Geometry check sheet. Reference: the model listing, model coordinates, mm. Coordinates: 2 decimals unless noted, no trailing zeros. Order: outer loops, then holes, each group sorted by start corner. A loop starts at its lowest first (then second) coordinate and runs counter-clockwise, first axis right, second up. Notation, with made-up numbers: (-33, 72.25) - (-13, 72.25) arc R16 ccw to (-13, 101.25) - close; hole circle Ø8 at (-6, 27). An arc over 180 degrees is marked (long way). Return JSON: item names as keys, results as strings. Group by question number.
Item 1: Scan lines: probe 1 along Y at (x, z) = (41, -2); probe 2 along Y at (x, z) = (-62, 0.25); probe 3 along X at (y, z) = (-2.5, 1.5). Record each from-to range of solid material in increasing order.
Item 2: Draft check along X on faces 1 (the conical face through (-23.88, -0.56, 4.27)), 2 (the conical face through (37.715, 3.943, 1.242)), 3 (the flat face through (-76.2, 0, 0)). Enter one of: pulls with the +X half, pulls with the -X half, needs draft (parallel to the pull), parting line crosses it, or undercut.
Item 3: Section check A-A on x = -63. Enter the section's corners in (y, z) (1 decimal).
Item 4: Gauge pin test, flat ends, axial feed: pin 1 (2 mm diameter, centred on x = 5, y = 2, fed in from +Z); pin 2 (2 mm diameter, centred on x = -4.5, z = -0.5, fed in from +Y); pin 3 (3 mm diameter, centred on y = -2.5, z = 3.5, fed in from +X). Record the tip position at first contact, or that the pin passes through.
Item 5: Section check B-B on x = 21. Enter the section's corners in (y, z) (1 decimal), then the cut area to 3 significant figures.
from build123d import *

# Parameters (mm, degrees)
F2_R = 2.54
F3_R = 1.27


with BuildPart() as f1:
    # F0 (on Top) → F1 (revolve)
    with BuildSketch(Plane.XY):
        with BuildLine():
            Line((-58.079902, 4.7625), (-76.2, 4.7625))
            Line((-76.2, 4.7625), (-76.2, 0))
            Line((-76.2, 0), (76.2, 0))
            Line((76.2, 0), (76.2, 3.4925))
            Line((76.2, 3.4925), (2.721047, 4.717149))
            ThreePointArc((2.721047, 4.717149), (2.9e-05, 4.738204), (-2.720931, 4.710673))
            Line((-2.720931, 4.710673), (-44.45, 3.915833))
            ThreePointArc((-44.45, 3.915833), (-50.389272, 4.03983), (-56.299735, 4.637118))
            ThreePointArc((-56.299735, 4.637118), (-57.187613, 4.731116), (-58.079902, 4.7625))
        make_face()
    revolve(axis=Axis((0, 0, 0), (1, 0, 0)))

    # F2
    f2_edges = [f1.edges().sort_by_distance(p)[0] for p in [
        (76.2, -3.4925, 0),
    ]]
    fillet(f2_edges, radius=F2_R)

    # F3
    f3_edges = [f1.edges().sort_by_distance(p)[0] for p in [
        (-76.2, -4.7625, 0),
    ]]
    fillet(f3_edges, radius=F3_R)


solid = f1.part
Computed:
{
 "1": {"probe 1": "y = -3.56 to 3.56", "probe 2": "y = -4.76 to 4.76", "probe 3": "x = -76.2 to 75.32"},
 "2": {"face 1": "undercut", "face 2": "pulls with the +X half", "face 3": "pulls with the -X half"},
 "3": {"outline": "circle Ø9.5 at (0, 0)"},
 "4": {"pin 1": "stops at z = 4.57", "pin 2": "stops at y = 4.69", "pin 3": "stops at x = 75.45"},
 "5": {"outline": "circle Ø8.8 at (0, 0)", "area": "61.2 mm²"}
}
